Part model, mm, in its own coordinate system. Face numbers are marked on the shaded views. A direction names the side the tool comes from. Round coordinates to 2 decimals unless told otherwise and drop trailing zeros. Write each loop counter-clockwise with the first axis right and the second up, starting at its lowest first coordinate (ties: lowest second). Pieces come first, ordered by that corner, then holes.
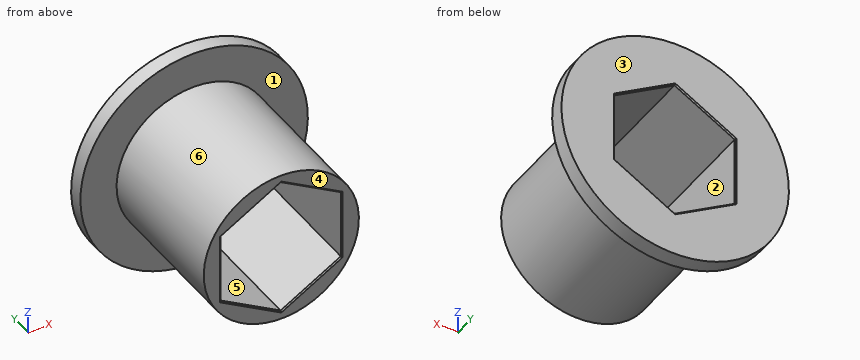
```python
from build123d import *

# Parameters (mm, degrees)
SKETCH1_R           = 6.35
BOSS_EXTRUDE1_DEPTH = 11.8872
SKETCH2_R           = 9.308550363
BOSS_EXTRUDE2_DEPTH = 1.27
CHAMFER1_SIZE       = 0.1
CHAMFER2_SIZE       = 0.1


with BuildPart() as part:
    # Sketch1 → Boss-Extrude1 (new body)
    with BuildSketch(Plane(origin=(0, 0, 0), x_dir=(1, 0, 0), z_dir=(0, 1, 0))):
        with Locations(Location((0, 0, 0), (0, 0, 270))):
            Circle(SKETCH1_R)
        Polygon((0, 5.689786881), (-4.927499981, 2.84489344), (-4.927499981, -2.84489344), (0, -5.689786881), (4.927499981, -2.84489344), (4.927499981, 2.84489344), align=None, mode=Mode.SUBTRACT)
    extrude(amount=BOSS_EXTRUDE1_DEPTH)

    # Sketch2 → Boss-Extrude2 (add)
    with BuildSketch(Plane(origin=(0, 11.8872, 0), x_dir=(1, 0, 0), z_dir=(0, 1, 0))):
        with Locations(Location((0, 0, 0), (0, 0, 270))):
            Circle(SKETCH2_R)
        Polygon((0, 5.689786881), (-4.927499981, 2.84489344), (-4.927499981, -2.84489344), (0, -5.689786881), (4.927499981, -2.84489344), (4.927499981, 2.84489344), align=None, mode=Mode.SUBTRACT)
    extrude(amount=BOSS_EXTRUDE2_DEPTH)

    # Chamfer1
    chamfer1_edges = [part.edges().sort_by_distance(p)[0] for p in [
        (-4.927499981, 0, 0),
        (-2.46374999, 0, 4.267340161),
        (2.463749991, 0, 4.267340161),
        (4.927499981, 0, 0),
        (2.46374999, 0, -4.267340161),
        (-2.463749991, 0, -4.267340161),
    ]]
    chamfer(chamfer1_edges, length=CHAMFER1_SIZE)

    # Chamfer2
    chamfer2_edges = [part.edges().sort_by_distance(p)[0] for p in [
        (2.46374999, 13.1572, -4.267340161),
        (-2.463749991, 13.1572, -4.267340161),
        (-4.927499981, 13.1572, 0),
        (-2.46374999, 13.1572, 4.267340161),
        (2.463749991, 13.1572, 4.267340161),
        (4.927499981, 13.1572, 0),
    ]]
    chamfer(chamfer2_edges, length=CHAMFER2_SIZE)


solid = part.part
```
Q1. Cut at D-D on x = 6. Write the cut outline in (y, z).
Values follow:
outline: (0, -2.08) - (11.89, -2.08) - (11.89, -7.12) - (13.16, -7.12) - (13.16, 7.12) - (11.89, 7.12) - (11.89, 2.08) - (0, 2.08) - close
Q2. Cut at C-C on y = 11. Write the cut outline in (x, z).
Values follow:
outline: circle Ø12.7 at (0, 0); hole (-4.93, -2.84) - (0, -5.69) - (4.93, -2.84) - (4.93, 2.84) - (0, 5.69) - (-4.93, 2.84) - close
Q3. Drop flat-ended pins along their axis: pin 1 (6.5 mm diameter, centred on y = 4.5, z = 0, fed in from -X); pin 2 (3 mm diameter, centred on y = 5.5, z = 0, fed in from +X); pin 3 (6 mm diameter, centred on y = 2, z = -6.5, fed in from +X); pin 4 (4 mm diameter, centred on x = 3, z = -2, fed in from -Y). Give the stop position or say it passes through.
Values follow:
pin 1: stops at x = -6.35
pin 2: stops at x = 6.35
pin 3: stops at x = 5.3
pin 4: stops at y = 0
Q4. Mould opens along Z. For the marked faces 4, 5 and 6 say: +Z half, -Z half, draft (parallel to the pull), parting line (faces both ways), or undercut.
Values follow:
face 4: draft
face 5: undercut
face 6: parting line
Q5. Wall check: L1, parallel to Y at x = -7.5, z = -4; L2, parallel to Z at x = 2.75, y = 5.75; L3, parallel to Z at x = 4, y = 4.5. Give the ranges that are in metal, low to high.
Values follow:
L1: y = 11.89 to 13.16
L2: z = -5.72 to -4.1, 4.1 to 5.72
L3: z = -4.93 to -3.38, 3.38 to 4.93
Q6. Cut at A-A on z = 0. Write the cut outline in (x, y).
Values follow:
outline: (-9.31, 11.89) - (-6.35, 11.89) - (-6.35, 0) - (-5.03, 0) - (-4.93, 0.1) - (-4.93, 13.06) - (-5.03, 13.16) - (-9.31, 13.16) - close; (4.93, 0.1) - (5.03, 0) - (6.35, 0) - (6.35, 11.89) - (9.31, 11.89) - (9.31, 13.16) - (5.03, 13.16) - (4.93, 13.06) - close
Q7. Cut at B-B on x = -0.25. Write the cut outline in (y, z).
Values follow:
outline: (0, -6.35) - (11.89, -6.35) - (11.89, -9.31) - (13.16, -9.31) - (13.16, -5.66) - (13.06, -5.55) - (0.1, -5.55) - (0, -5.66) - close; (0, 5.66) - (0.1, 5.55) - (13.06, 5.55) - (13.16, 5.66) - (13.16, 9.31) - (11.89, 9.31) - (11.89, 6.35) - (0, 6.35) - close
Q8. Which spindle directions (+Z, -Z, +X, -X, +Y, -Y) get a long thin tool onto all of the face, cutting with end or side? Do the marked faces 1, 2 and 3. Say none if no direction does.
Values follow:
face 1: -Y
face 2: +Y, -Y
face 3: +Z, -Z, +X, -X, +Y
